```python
from build123d import *

# Parameters (mm, degrees)
PAD_DEPTH     = 2
SKETCH001_R   = 1.75
POCKET_DEPTH  = 5
SKETCH002_R   = 3
SKETCH002_R_2 = 1.6
PAD001_DEPTH  = 21


with BuildPart() as part:
    # Sketch → Pad (new body)
    with BuildSketch(Plane.XY):
        with BuildLine():
            Line((-25.000066, 40.999736), (24.999953, 40.999736))
            ThreePointArc((28.000009, 38.000002), (27.121199, 40.121154), (24.999953, 40.999736))
            Line((28.000009, 38.000002), (28.000116, 37))
            ThreePointArc((25.000438, 34), (27.121645, 34.878699), (28.000116, 37))
            Line((25.000438, 34), (23, 34))
            ThreePointArc((23, 34), (22.292893, 33.707107), (22, 33))
            Line((22, 33), (22, -1.000001))
            ThreePointArc((22, -1.000001), (22.292893, -1.707108), (23, -2.000001))
            Line((23, -2.000001), (26.999998, -2.000001))
            ThreePointArc((27.999996, -2.999999), (27.707103, -2.292894), (26.999998, -2.000001))
            Line((27.999996, -2.999999), (27.999996, -21.999992))
            ThreePointArc((25.000004, -24.999984), (27.121319, -24.121306), (27.999996, -21.999992))
            Line((25.000004, -24.999984), (-24.999967, -24.999984))
            ThreePointArc((-27.999934, -22.000016), (-27.121264, -24.121314), (-24.999967, -24.999984))
            Line((-27.999934, -22.000016), (-27.999934, 37.999868))
            ThreePointArc((-25.000066, 40.999736), (-27.121293, 40.121095), (-27.999934, 37.999868))
        make_face()
    extrude(amount=-PAD_DEPTH)

    # Sketch001 (on Face16 of Pad) → Pocket (cut)
    with BuildSketch(Plane.XY):
        with Locations((-8.896551, 37.535175)):
            Circle(SKETCH001_R)
        with Locations((19.048174, 37.554218)):
            Circle(SKETCH001_R)
        with Locations((-24.112202, -13.254919)):
            Circle(SKETCH001_R)
        with Locations((24.153093, -14.517437)):
            Circle(SKETCH001_R)
    extrude(amount=-POCKET_DEPTH, mode=Mode.SUBTRACT)

    # Sketch002 (on Face5 of Pocket) → Pad001 (join)
    with BuildSketch(Plane(origin=(0, 0, -2), x_dir=(1, 0, 0), z_dir=(0, 0, -1))):
        with Locations((-24.440964, 20.497406)):
            Circle(SKETCH002_R)
        with Locations((-24.440964, 20.497406)):
            Circle(SKETCH002_R_2, mode=Mode.SUBTRACT)
        with Locations((24.491911, 20.496445)):
            Circle(SKETCH002_R)
        with Locations((24.491911, 20.496445)):
            Circle(SKETCH002_R_2, mode=Mode.SUBTRACT)
        with Locations((-24.511511, -37.516029)):
            Circle(SKETCH002_R)
        with Locations((-24.511511, -37.516029)):
            Circle(SKETCH002_R_2, mode=Mode.SUBTRACT)
        with Locations((24.504074, -37.505135)):
            Circle(SKETCH002_R)
        with Locations((24.504074, -37.505135)):
            Circle(SKETCH002_R_2, mode=Mode.SUBTRACT)
    extrude(amount=PAD001_DEPTH)


with BuildPart() as part_1:
    # Body placement: moved
    add(part.part.moved(Location((0, 0, 24.5))))


with BuildPart() as part_2:
    # Clone placement: moved
    add(part_1.part.moved(Location((0, 0, 55.5))))


solid = part_2.part
```
Geometry check sheet. Reference: the model listing, model coordinates, mm. A direction names the side the tool comes from. Round coordinates to 2 decimals unless told otherwise and drop trailing zeros. Loops run counter-clockwise (first coordinate to the right, second up) from the corner with the lowest first, then second, coordinate; pieces in that order, holes last. Notation, with made-up numbers: (7.25, 15) - (62.25, 15) arc R20 ccw to (62.25, 39) - close; hole circle Ø5 at (54.5, -32). An arc over 180 degrees is marked (long way). Use a Markdown table: item, result.
Q1. Material ranges on line 1 (X direction, y = -20.5, z = 66.5); line 2 (X direction, y = -21, z = 58.5); line 3 (Y direction, x = -25.5, z = 63.75), recorded low to high.
Solutions:
| item | result |
|---|---|
| line 1 | x = -27.44 to -26.04, -22.84 to -21.44, 21.49 to 22.89, 26.09 to 27.49 |
| line 2 | x = -27.4 to -25.96, -22.92 to -21.48, 21.53 to 22.97, 26.01 to 27.45 |
| line 3 | y = -23.3 to -21.7, -19.3 to -17.69, 34.68 to 36.26, 38.77 to 40.35 |
Q2. Access from +Z, -Z, +X, -X, +Y, -Y to the whole of each face (thin tool, end or side, straight path). Record for faces 1 (the flat face through (-23, 39, 57)), 2 (the cylindrical face through (23.325, 36.424, 67.647)), 3 (the cylindrical face through (27.1, 34.86, 79.01)).
Solutions:
| item | result |
|---|---|
| face 1 | -Z, +X, -X, +Y, -Y |
| face 2 | -Z |
| face 3 | +Z, -Z, +X |
Q3. Cross-section at A-A on z = 71.75. Record the cut outline in (x, y), plus the area to 3 significant figures.
Solutions:
| item | result |
|---|---|
| outline | circle Ø6 at (-24.51, 37.52); circle Ø6 at (-24.44, -20.5); circle Ø6 at (24.49, -20.5); circle Ø6 at (24.5, 37.51); hole circle Ø3.2 at (-24.51, 37.52); hole circle Ø3.2 at (-24.44, -20.5); hole circle Ø3.2 at (24.49, -20.5); hole circle Ø3.2 at (24.5, 37.51) |
| area | 80.9 mm2 |
Q4. Cross-section at B-B on x = -8.5. Record the cut outline in (y, z), plus the area to 3 significant figures.
Solutions:
| item | result |
|---|---|
| outline | (-25, 78) - (35.83, 78) - (35.83, 80) - (-25, 80) - close; (39.24, 78) - (41, 78) - (41, 80) - (39.24, 80) - close |
| area | 125 mm2 |
Q5. Cross-section at C-C on x = -1. Record the cut outline in (y, z), plus the area to 3 significant figures.
Solutions:
| item | result |
|---|---|
| outline | (-25, 78) - (41, 78) - (41, 80) - (-25, 80) - close |
| area | 132 mm2 |
Q6. Draft check along Y on faces 4 (the cylindrical face through (22.29, 35.48, 67.65)), 5 (the cylindrical face through (-27.1, 40.14, 79.01)), 6 (the flat face through (-23, -19, 57)). Enter one of: released by +Y, released by -Y, zero draft, split by the parting line, or undercut.
Solutions:
| item | result |
|---|---|
| face 4 | undercut |
| face 5 | released by +Y |
| face 6 | zero draft |
Q7. Go/stop test with flat-tipped pins: P1, Ø6, axis at x = -7.5, y = -3, coming from the -Z side; P2, Ø1, axis at y = 21.5, z = 79.5, coming from the +X side. Record where each tip stops, or that it passes through.
Solutions:
| item | result |
|---|---|
| P1 | stops at z = 78 |
| P2 | stops at x = 22 |
Q8. Cross-section at D-D on y = -9.5. Record the cut outline in (x, z).
Solutions:
| item | result |
|---|---|
| outline | (-28, 78) - (28, 78) - (28, 80) - (-28, 80) - close |
